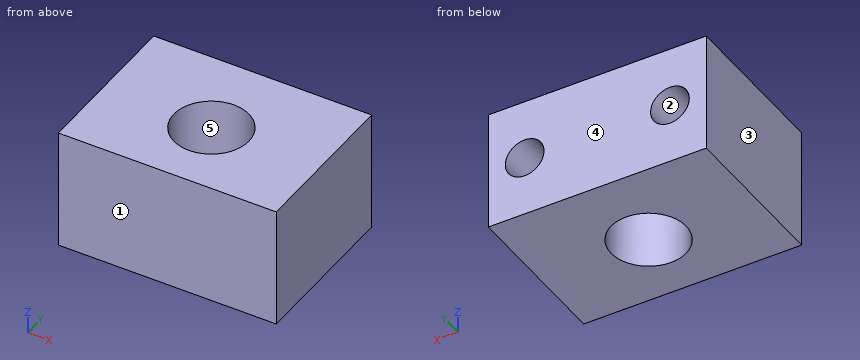
```python
from build123d import *

# Parameters (mm, degrees)
SKETCH_1_W          = 18
SKETCH_1_H          = 13.2
SKETCH_1_R          = 3.1
EXTRUDE_1_DEPTH     = 10
SKETCH_2_R          = 1.6
CUT_EXTRUDE_1_DEPTH = 10


with BuildPart() as part:
    # ｽｹｯﾁ1 → ﾎﾞｽ - 押し出し1 (new body)
    with BuildSketch(Plane.XY):
        with Locations((0, 0.5)):
            Rectangle(SKETCH_1_W, SKETCH_1_H)
        Circle(SKETCH_1_R, mode=Mode.SUBTRACT)
    extrude(amount=EXTRUDE_1_DEPTH)

    # ｽｹｯﾁ2 → ｶｯﾄ - 押し出し1 (cut)
    with BuildSketch(Plane(origin=(0, 7.1, 0), x_dir=(1, 0, 0), z_dir=(0, 1, 0))):
        with Locations(Location((-6, -5, 0), (0, 0, 180))):
            Circle(SKETCH_2_R)
        with Locations((6, -5)):
            Circle(SKETCH_2_R)
    extrude(amount=-CUT_EXTRUDE_1_DEPTH, mode=Mode.SUBTRACT)


solid = part.part
```
The model under review builds one solid part; all positions refer to its coordinate system, in mm. Face numbers are marked on the shaded views. A direction names the side the tool comes from. Round coordinates to 2 decimals unless told otherwise and drop trailing zeros. Order: outer loops, then holes, each group sorted by start corner. A loop starts at its lowest first (then second) coordinate and runs counter-clockwise, first axis right, second up. Notation, with made-up numbers: (32.25, -38.75) -> (79.25, -38.75) arc R24 ccw to (79.25, -10.75) -> close; hole circle Ø3 at (30, 11). An arc over 180 degrees is marked (long way). Use a Markdown table: item, result.
Q1. Clearance check with a flat-ended pin moving along its axis: P1, Ø1, axis at x = 6.5, z = 5.5, coming from the +Y side. State where the tip first meets the part, or that it passes through.
Values:
| item | result |
|---|---|
| P1 | stops at y = -2.9 |
Q2. Tool access review of the marked faces 1 and 2: name each direction out of +Z, -Z, +X, -X, +Y, -Y from which nothing blocks a thin tool from reaching the whole face with its end or side.
Values:
| item | result |
|---|---|
| face 1 | +Z, -Z, +X, -X, -Y |
| face 2 | +Y |
Q3. We need section A-A on x = 0. Write out the cut boundary in (y, z), then the cut area to 3 significant figures.
Values:
| item | result |
|---|---|
| outline | (-6.1, 0) -> (-3.1, 0) -> (-3.1, 10) -> (-6.1, 10) -> close; (3.1, 0) -> (7.1, 0) -> (7.1, 10) -> (3.1, 10) -> close |
| area | 70.0 mm^2 |
Q4. For line 1 (Z direction, x = -6, y = 1.5); line 2 (Y direction, x = 0, z = 5.25); line 3 (X direction, y = -1.75, z = 4.75), list the stretches that pass through material, from the lowest coordinate up.
Values:
| item | result |
|---|---|
| line 1 | z = 0 to 3.4, 6.6 to 10 |
| line 2 | y = -6.1 to -3.1, 3.1 to 7.1 |
| line 3 | x = -9 to -7.58, -4.42 to -2.56, 2.56 to 4.42, 7.58 to 9 |
Q5. We need section B-B on z = 5. Write out the cut boundary in (x, y), then the cut area to 3 significant figures.
Values:
| item | result |
|---|---|
| outline | (-9, -6.1) -> (9, -6.1) -> (9, 7.1) -> (7.6, 7.1) -> (7.6, -2.9) -> (4.4, -2.9) -> (4.4, 7.1) -> (-4.4, 7.1) -> (-4.4, -2.9) -> (-7.6, -2.9) -> (-7.6, 7.1) -> (-9, 7.1) -> close; hole circle Ø6.2 at (0, 0) |
| area | 143 mm^2 |
Q6. Mouldability with a two-part tool opening along X and no side actions: class the marked faces 3, 4 and 5 as +X half, -X half, draft (parallel to the pull), parting line (faces both ways), or undercut.
Values:
| item | result |
|---|---|
| face 3 | -X half |
| face 4 | draft |
| face 5 | undercut |
Q7. We need section C-C on y = 0.5. Write out the cut boundary in (x, z).
Values:
| item | result |
|---|---|
| outline | (-9, 0) -> (-3.06, 0) -> (-3.06, 10) -> (-9, 10) -> close; (3.06, 0) -> (9, 0) -> (9, 10) -> (3.06, 10) -> close; hole circle Ø3.2 at (-6, 5); hole circle Ø3.2 at (6, 5) |
Q8. We need section D-D on y = 5.25. Write out the cut boundary in (x, z), then the cut area to 3 significant figures.
Values:
| item | result |
|---|---|
| outline | (-9, 0) -> (9, 0) -> (9, 10) -> (-9, 10) -> close; hole circle Ø3.2 at (-6, 5); hole circle Ø3.2 at (6, 5) |
| area | 164 mm^2 |
